Autodesk Inventor part; units mm, degrees
ref_plane "YZ Plane" through (0, 0, 0) normal (1, 0, 0) x (0, 1, 0)
ref_plane "XZ Plane" through (0, 0, 0) normal (0, 1, 0) x (-1, 0, 0)
ref_plane "XY Plane" through (0, 0, 0) normal (0, 0, 1) x (1, 0, 0)
sketch "Sketch1" plane through (0, 0, 0) normal (0, 0, 1) x (1, 0, 0)
  line L0 (0, 4.2672) -> (0, -4.2672)
  line L1 (-5.7785, 0) -> (5.7785, 0)
  line L2 (4.1275, -3.048) -> (-4.1275, -3.048)
  line L3 (-4.1275, -3.048) -> (-4.1275, 3.048)
  line L4 (-4.1275, 3.048) -> (4.1275, 3.048)
  line L5 (4.1275, 3.048) -> (4.1275, -3.048)
  line L6 (4.1275, -3.048) -> (-4.1275, 3.048) construction
  line L7 (-4.1275, -3.048) -> (4.1275, 3.048) construction
  point P0 (0, 0)
  dimension "d0" = 8.255
  dimension "d1" = 6.096
extrude "Extrusion1" add sketch "Sketch1" along normal blind 0.9652
sketch "Sketch2" plane through (4.1275, -3.048, 0) normal (1, 0, 0) x (0, 0, -1)
  line L0 (0, 0) -> (-0.9652, 0)
  line L1 (-0.9652, 0) -> (-0.9652, 6.096)
  line L2 (0, 6.096) -> (0, 0)
  line L3 (-0.4572, 0) -> (-0.4572, 0.9474)
  line L4 (-0.4572, 0.9474) -> (-0.9652, 0.6541)
  line L5 (-0.9652, 0.6541) -> (-0.9652, 0)
  line L6 (-0.9652, 0) -> (-0.4572, 0)
  line L7 (-1.1582, 3.048) -> (0.193, 3.048)
  point P0 (0, 3.048)
  dimension "d4" = 0.508
  dimension "d5" = 0.9474
  dimension "d6" = 60
  dimension "d15" = 0.6541
  dimension "d16" = 2.1006
extrude "Extrusion2" cut sketch "Sketch2" against normal blind 8.255 contours L0 L1 L4 L3
mirror "Mirror1" about plane through (0, 0, 0) normal (0, 1, 0) of "Extrusion2"
sketch "Sketch4" plane through (0, 0, 0.9652) normal (0, 0, 1) x (1, 0, 0)
  line L0 (0, 4.2672) -> (0, -4.2672)
  line L1 (-5.7785, 0) -> (5.7785, 0)
  line L2 (-4.1275, 2.3939) -> (-4.1275, -2.3939)
  line L3 (4.1275, -1.2192) -> (-4.1275, -1.2192)
  line L4 (-4.1275, -1.2192) -> (-4.1275, 1.2192)
  line L5 (-4.1275, 1.2192) -> (4.1275, 1.2192)
  line L6 (4.1275, 1.2192) -> (4.1275, -1.2192)
  line L7 (4.1275, -1.2192) -> (-4.1275, 1.2192) construction
  line L8 (-4.1275, -1.2192) -> (4.1275, 1.2192) construction
  point P0 (0, 0)
  dimension "d17" = 2.4384
extrude "Extrusion4" [suppressed]
sketch "Sketch5" plane through (0, 0, 0) normal (1, 0, 0) x (0, 1, 0)
  line L0 (3.048, 0) -> (-3.048, 0)
  line L1 (-3.048, 0) -> (-3.048, 0.4572)
  line L2 (3.048, 0) -> (3.048, 0.4572)
  line L3 (-3.048, 0) -> (-2.7686, 0)
  line L4 (-2.7686, 0) -> (-2.7686, -0.4572)
  line L5 (-2.7686, -0.4572) -> (-3.048, -0.4572)
  line L6 (-3.048, -0.4572) -> (-3.048, 0)
  line L7 (3.048, 0) -> (2.7686, 0)
  line L8 (2.7686, 0) -> (2.7686, -0.4572)
  line L9 (2.7686, -0.4572) -> (3.048, -0.4572)
  line L10 (3.048, -0.4572) -> (3.048, 0)
  point P0 (0, 0)
  dimension "d20" = 0.4572
  dimension "d21" = 5.5372
extrude "Extrusion5" add sketch "Sketch5" against normal up to surface (8.255 mm away) from surface at 4.1275 contours L4 L5 L6 L0
properties part number "J007869" material "ALUMINUM, 6061-T651"
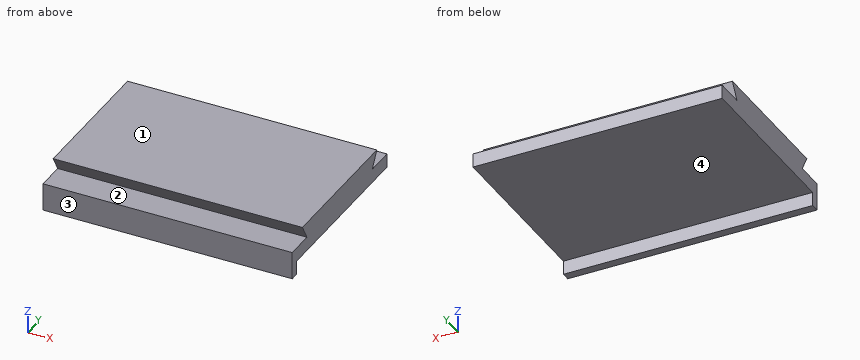
Verification items for the finished model (mm, model axes). Face numbers are marked on the shaded views. Give positions to 0.01 mm unless a question says otherwise; leave off trailing zeros. Order: outer loops, then holes, each group sorted by start corner. A loop starts at its lowest first (then second) coordinate and runs counter-clockwise, first axis right, second up. Notation, with made-up numbers: (-16.75, -20) - (29.25, -20) arc R29 cw to (29.25, 17) - close; hole circle Ø1 at (31, -33). An arc over 180 degrees is marked (long way). Answer as CSV lines item,"result". Start each with the question number.
Item 1: Section check B-B, the plane y = -2.25. Record the boundary of the cut face in (x, z).
Item 2: Section check A-A, the plane x = 0.25. Record the boundary of the cut face in (y, z), plus the area to 3 significant figures.
Item 3: Mould release check, pull along Z, two halves, no side actions. Record for the marked faces 1, 2, 3 and 4: released by +Z, released by -Z, zero draft, split by the parting line, or undercut.
Item 4: Material ranges on L1, parallel to Z at x = 0.5, y = 0.25; L2, parallel to Z at x = 1.25, y = 2.25; L3, parallel to Z at x = 1, y = 2.5, recorded low to high.
Item 5: Section check D-D, the plane z = -0.3. Record the boundary of the cut face in (x, y), plus the area to 3 significant figures.
Item 6: Section check C-C, the plane y = 2.75. Record the boundary of the cut face in (x, z).
Filled in:
1,outline,"(-4.13, 0) - (4.13, 0) - (4.13, 0.46) - (-4.13, 0.46) - close; (-4.13, 0.72) - (4.13, 0.72) - (4.13, 0.97) - (-4.13, 0.97) - close"
2,outline,"(-3.05, -0.46) - (-2.77, -0.46) - (-2.77, 0) - (3.05, 0) - (3.05, 0.46) - (2.1, 0.46) - (2.39, 0.97) - (-2.39, 0.97) - (-2.1, 0.46) - (-3.05, 0.46) - close"
2,area,"5.20 mm^2"
3,face 1,"released by +Z"
3,face 2,"undercut"
3,face 3,"zero draft"
3,face 4,"released by -Z"
4,L1,"0 to 0.97"
4,L2,"0 to 0.46, 0.72 to 0.97"
4,L3,"0 to 0.46"
5,outline,"(-4.13, -3.05) - (4.13, -3.05) - (4.13, -2.77) - (-4.13, -2.77) - close"
5,area,"2.31 mm^2"
6,outline,"(-4.13, 0) - (4.13, 0) - (4.13, 0.46) - (-4.13, 0.46) - close"
